Design review of the part built by this model. Coordinates are the model's own, in mm. A direction names the side the tool comes from. Give positions to 0.01 mm unless a question says otherwise; leave off trailing zeros. Write each loop counter-clockwise with the first axis right and the second up, starting at its lowest first coordinate (ties: lowest second). Pieces come first, ordered by that corner, then holes. Notation, with made-up numbers: (9.5, 83) -> (47.5, 83) arc R23 ccw to (47.5, 110) -> close; hole circle Ø6 at (32.25, 27). An arc over 180 degrees is marked (long way). Return JSON: item names as keys, results as strings. Group by question number.
from build123d import *

# Parameters (mm, degrees)
SKETCH002_W     = 135
SKETCH002_H     = 80
PAD_DEPTH       = 70
SKETCH003_W     = 128
SKETCH003_H     = 13
POCKET_DEPTH    = 64
SKETCH001_W     = 82
SKETCH001_H     = 52
POCKET001_DEPTH = 1
FILLET_R        = 10
FILLET001_R     = 2
FILLET002_R     = 15
FILLET003_R     = 20


with BuildPart() as part:
    # Sketch002 → Pad (new body)
    with BuildSketch(Plane.XY):
        with Locations((-0.5, -39.9)):
            Rectangle(SKETCH002_W, SKETCH002_H)
    extrude(amount=-PAD_DEPTH)

    # Sketch003 → Pocket (cut)
    with BuildSketch(Plane(origin=(0, 0.1, 0), x_dir=(-1, 0, 0), z_dir=(0, 1, 0))):
        with Locations((0, -7.5)):
            Rectangle(SKETCH003_W, SKETCH003_H)
    extrude(amount=-POCKET_DEPTH, mode=Mode.SUBTRACT)

    # Sketch001 → Pocket001 (cut)
    with BuildSketch(Plane.XY):
        with Locations((0, -32)):
            Rectangle(SKETCH001_W, SKETCH001_H)
    extrude(amount=-POCKET001_DEPTH, mode=Mode.SUBTRACT)

    # Fillet
    fillet_edges = [part.edges().sort_by_distance(p)[0] for p in [
        (-41, -58, -0.5),
        (41, -58, -0.5),
        (-41, -6, -0.5),
        (41, -6, -0.5),
    ]]
    fillet(fillet_edges, radius=FILLET_R)

    # Fillet001
    fillet001_edges = [part.edges().sort_by_distance(p)[0] for p in [
        (-68, 0.1, -35),
        (67, 0.1, -35),
    ]]
    fillet(fillet001_edges, radius=FILLET001_R)

    # Fillet002
    fillet002_edges = [part.edges().sort_by_distance(p)[0] for p in [
        (67, -79.9, -35),
        (-68, -79.9, -35),
    ]]
    fillet(fillet002_edges, radius=FILLET002_R)

    # Fillet003
    fillet003_edges = [part.edges().sort_by_distance(p)[0] for p in [
        (-0.5, -79.9, -70),
        (-0.5, 0.1, -70),
    ]]
    fillet(fillet003_edges, radius=FILLET003_R)


solid = part.part
Q1. For L1, parallel to Z at x = 43.5, y = -48; L2, parallel to X at y = -65.5, z = -47; L3, parallel to X at y = -59, z = -4.5, list the stretches that pass through material, from the lowest coordinate up. Write a range as from..to.
Q2. Tool access review of faces 1 (the face through (-62.297, -33.841, -63.986)), 2 (the face through (1, -60, -1)), 3 (the face through (61.297, -32.959, -63.986)): name each direction out of +Z, -Z, +X, -X, +Y, -Y from which nothing blocks a thin tool from reaching the whole face with its end or side.
Q3. Take a section at B-B, the plane z = -5. Give the boundary of the cut face in (x, y).
Q4. Take a section at A-A, the plane x = -0.5. Give the boundary of the cut face in (y, z), plus the area to 3 significant figures.
Q5. Take a section at C-C, the plane y = -39.5. Give the boundary of the cut face in (x, z).
Q6. Insertion check: pin 1 (8 mm diameter, centred on y = -42, z = -55.5, fed in from -X); pin 2 (5 mm diameter, centred on x = 32, y = -14.5, fed in from +Z); pin 3 (6.5 mm diameter, centred on x = 31, z = -8.5, fed in from +Y). Each pin has a flat end and moves straight along its axis. Give the tip position at first contact, or say it passes through.
Q7. Mouldability with a two-part tool opening along X and no side actions: class faces 4 (the face through (-1.417, -5.603, -63.986)), 5 (the face through (67, -34, -25)), 6 (the face through (-1, -66, 0)) as +X half, -X half, draft (parallel to the pull), parting line (faces both ways), or undercut.
Q8. Take a section at D-D, the plane x = 32.5. Give the boundary of the cut face in (y, z).
Final values:
{
 "1": {"L1": "z = -70..-14, -1..0", "L2": "x = -67.99..66.99", "L3": "x = -68..-64, 64..67"},
 "2": {"face 1": "-Z, -X, -Y", "face 2": "+Y", "face 3": "-Z, +X, -Y"},
 "3": {"outline": "(-68, -64.9) arc R15 ccw to (-53, -79.9) -> (52, -79.9) arc R15 ccw to (67, -64.9) -> (67, -1.9) arc R2 ccw to (65, 0.1) -> (64, 0.1) -> (64, -63.9) -> (-64, -63.9) -> (-64, 0.1) -> (-66, 0.1) arc R2 ccw to (-68, -1.9) -> close"},
 "4": {"outline": "(-79.9, -50) arc R20 ccw to (-59.9, -70) -> (-19.9, -70) arc R20 ccw to (0.1, -50) -> (0.1, -14) -> (-63.9, -14) -> (-63.9, -1) -> (-58, -1) -> (-58, 0) -> (-79.9, 0) -> close; (-6, -1) -> (0.1, -1) -> (0.1, 0) -> (-6, 0) -> close", "area": "4,540 mm²"},
 "5": {"outline": "(-68, -50) arc R20 ccw to (-48, -70) -> (47, -70) arc R20 ccw to (67, -50) -> (67, 0) -> (41, 0) -> (41, -1) -> (64, -1) -> (64, -14) -> (-64, -14) -> (-64, -1) -> (-41, -1) -> (-41, 0) -> (-68, 0) -> close"},
 "6": {"pin 1": "stops at x = -67.94", "pin 2": "stops at z = -14", "pin 3": "stops at y = -63.9"},
 "7": {"face 4": "undercut", "face 5": "+X half", "face 6": "draft"},
 "8": {"outline": "(-79.9, -50) arc R20 ccw to (-59.9, -70) -> (-19.9, -70) arc R20 ccw to (0.1, -50) -> (0.1, -14) -> (-63.9, -14) -> (-63.9, -1) -> (-57.89, -1) -> (-57.89, 0) -> (-79.9, 0) -> close; (-6.11, -1) -> (0.1, -1) -> (0.1, 0) -> (-6.11, 0) -> close"}
}
